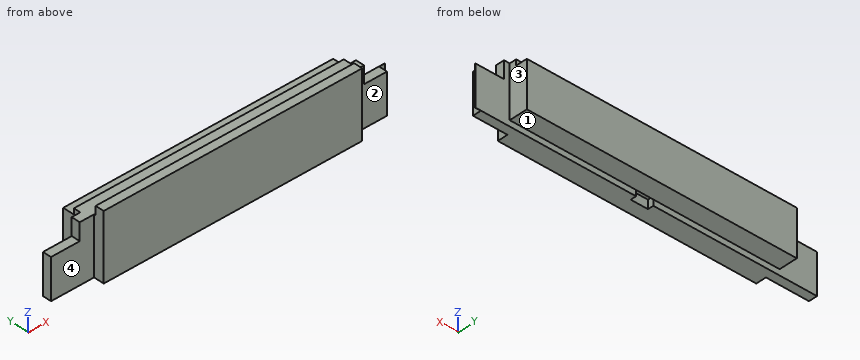
from build123d import *

# Parameters (mm, degrees)
SKETCH042_W     = 610
SKETCH042_H     = 115
PAD004_DEPTH    = 65
SKETCH043_W     = 60
SKETCH043_H     = 32
SKETCH043_W_2   = 70
SKETCH043_H_2   = 18
POCKET037_DEPTH = 115.001
SKETCH044_W     = 80
SKETCH044_H     = 32
SKETCH044_W_2   = 90
SKETCH044_H_2   = 18
POCKET038_DEPTH = 115.001
SKETCH045_W     = 50
SKETCH045_H     = 45
POCKET039_DEPTH = 65.001
SKETCH046_W     = 65
SKETCH046_H     = 45
POCKET040_DEPTH = 65.001
SKETCH047_W     = 30
SKETCH047_H     = 10
POCKET041_DEPTH = 15
SKETCH048_W     = 610
SKETCH048_H     = 32
POCKET042_DEPTH = 10
SKETCH049_W     = 20
SKETCH049_H     = 25
POCKET043_DEPTH = 610.001
SKETCH050_W     = 50
SKETCH050_H     = 15
POCKET044_DEPTH = 610.001
SKETCH051_W     = 15
SKETCH051_H     = 65
POCKET045_DEPTH = 115.001
SKETCH052_W     = 10
SKETCH052_H     = 32.5
POCKET046_DEPTH = 115.001


with BuildPart() as part:
    # Sketch042 (on DatumPlane) → Pad004 (new body)
    with BuildSketch(Plane.XZ.offset(32.5)):
        Rectangle(SKETCH042_W, SKETCH042_H)
    extrude(amount=-PAD004_DEPTH)

    # Sketch043 (on DatumPlane) → Pocket037 (cut, through all)
    with BuildSketch(Plane.XY.offset(57.5)):
        with Locations((275, 16.5)):
            Rectangle(SKETCH043_W, SKETCH043_H)
        with Locations((270, -23.5)):
            Rectangle(SKETCH043_W_2, SKETCH043_H_2)
    extrude(amount=-POCKET037_DEPTH, mode=Mode.SUBTRACT)

    # Sketch044 (on DatumPlane) → Pocket038 (cut, through all)
    with BuildSketch(Plane.XY.offset(57.5)):
        with Locations((-265, 16.5)):
            Rectangle(SKETCH044_W, SKETCH044_H)
        with Locations((-260, -23.5)):
            Rectangle(SKETCH044_W_2, SKETCH044_H_2)
    extrude(amount=-POCKET038_DEPTH, mode=Mode.SUBTRACT)

    # Sketch045 (on DatumPlane) → Pocket039 (cut, through all)
    with BuildSketch(Plane.XZ.offset(32.5)):
        with Locations((280, 35)):
            Rectangle(SKETCH045_W, SKETCH045_H)
    extrude(amount=-POCKET039_DEPTH, mode=Mode.SUBTRACT)

    # Sketch046 (on DatumPlane) → Pocket040 (cut, through all)
    with BuildSketch(Plane.XZ.offset(32.5)):
        with Locations((-272.5, 35)):
            Rectangle(SKETCH046_W, SKETCH046_H)
    extrude(amount=-POCKET040_DEPTH, mode=Mode.SUBTRACT)

    # Sketch047 (on DatumPlane) → Pocket041 (cut)
    with BuildSketch(Plane(origin=(0, 0, -57.5), x_dir=(-1, 0, 0), z_dir=(0, 0, -1))):
        with Locations((-10, -4.5)):
            Rectangle(SKETCH047_W, SKETCH047_H)
    extrude(amount=-POCKET041_DEPTH, mode=Mode.SUBTRACT)

    # Sketch048 (on DatumPlane) → Pocket042 (cut)
    with BuildSketch(Plane(origin=(0, 0, -57.5), x_dir=(-1, 0, 0), z_dir=(0, 0, -1))):
        with Locations((0, 16.5)):
            Rectangle(SKETCH048_W, SKETCH048_H)
    extrude(amount=-POCKET042_DEPTH, mode=Mode.SUBTRACT)

    # Sketch049 (on DatumPlane) → Pocket043 (cut, through all)
    with BuildSketch(Plane.YZ.offset(305)):
        with Locations((22.5, 45)):
            Rectangle(SKETCH049_W, SKETCH049_H)
    extrude(amount=-POCKET043_DEPTH, mode=Mode.SUBTRACT)

    # Sketch050 (on DatumPlane) → Pocket044 (cut, through all)
    with BuildSketch(Plane.YZ.offset(305)):
        with Locations((7.5, 50)):
            Rectangle(SKETCH050_W, SKETCH050_H)
    extrude(amount=-POCKET044_DEPTH, mode=Mode.SUBTRACT)

    # Sketch051 (on DatumPlane) → Pocket045 (cut, through all)
    with BuildSketch(Plane.XY.offset(57.5)):
        with Locations((-297.5, 0)):
            Rectangle(SKETCH051_W, SKETCH051_H)
    extrude(amount=-POCKET045_DEPTH, mode=Mode.SUBTRACT)

    # Sketch052 (on DatumPlane) → Pocket046 (cut, through all)
    with BuildSketch(Plane.XY.offset(57.5)):
        with Locations((300, -16.25)):
            Rectangle(SKETCH052_W, SKETCH052_H)
    extrude(amount=-POCKET046_DEPTH, mode=Mode.SUBTRACT)


solid = part.part
Can you work these out from the model? Positions are in its coordinate system, mm. Face numbers are marked on the shaded views. A direction names the side the tool comes from. Give positions to 0.01 mm unless a question says otherwise; leave off trailing zeros. Loops run counter-clockwise (first coordinate to the right, second up) from the corner with the lowest first, then second, coordinate; pieces in that order, holes last. Notation, with made-up numbers: (33.5, 6.25) -> (45.5, 6.25) arc R9 ccw to (45.5, 21.25) -> close; hole circle Ø7 at (25, 4.25). An arc over 180 degrees is marked (long way). Write item = value, one per line.
1) Will these pins go through, and if not, where does the flat tip stop? pin 1 (4 mm diameter, centred on x = -219.5, y = 21.5, fed in from -Z); pin 2 (5 mm diameter, centred on x = 13, y = -4, fed in from -Z); pin 3 (14.5 mm diameter, centred on y = -25, z = 6, fed in from +X).
Check result:
pin_1 = -47.5
pin_2 = -42.5
pin_3 = 235
2) Suppose I cut it at C-C on x = 6.5. Write out the boundary of the cut face in (y, z), then the cut area to 4 significant figures.
Check result:
outline = (-32.5, -57.5) -> (-9.5, -57.5) -> (-9.5, -42.5) -> (0.5, -42.5) -> (0.5, -47.5) -> (32.5, -47.5) -> (32.5, 32.5) -> (12.5, 32.5) -> (12.5, 42.5) -> (-17.5, 42.5) -> (-17.5, 57.5) -> (-32.5, 57.5) -> close
area = 6,055 mm2
3) Suppose I cut it at D-D on z = 27. Write out the boundary of the cut face in (x, y), then the cut area to 3 significant figures.
Check result:
outline = (-240, -14.5) -> (-215, -14.5) -> (-215, -32.5) -> (235, -32.5) -> (235, -14.5) -> (255, -14.5) -> (255, 0.5) -> (245, 0.5) -> (245, 32.5) -> (-225, 32.5) -> (-225, 0.5) -> (-240, 0.5) -> close
area = 30,600 mm2
4) Suppose I cut it at B-B on x = -73. Write out the boundary of the cut face in (y, z).
Check result:
outline = (-32.5, -57.5) -> (0.5, -57.5) -> (0.5, -47.5) -> (32.5, -47.5) -> (32.5, 32.5) -> (12.5, 32.5) -> (12.5, 42.5) -> (-17.5, 42.5) -> (-17.5, 57.5) -> (-32.5, 57.5) -> close
5) For the marked faces 1, 2, 3 and 4, which set-ups out of +Z, -Z, +X, -X, +Y, -Y let a thin tool reach every point of the face, with its end or its side?
Check result:
face_1 = -Z, +X, -X, +Y
face_2 = +Z, -Z, +X, -Y
face_3 = +Z, -Z, +X, +Y
face_4 = +Z, -Z, -X, -Y
6) Suppose I cut it at A-A on z = 2.5. Write out the boundary of the cut face in (x, y), then the cut area to 3 significant figures.
Check result:
outline = (-290, -14.5) -> (-215, -14.5) -> (-215, -32.5) -> (235, -32.5) -> (235, -14.5) -> (295, -14.5) -> (295, 0) -> (305, 0) -> (305, 0.5) -> (245, 0.5) -> (245, 32.5) -> (-225, 32.5) -> (-225, 0.5) -> (-290, 0.5) -> close
area = 31,900 mm2
7) I need wall thicknesses on L1, parallel to X at y = -3, z = -46.5; L2, parallel to Y at x = 203, z = 51; L3, parallel to X at y = 26.5, z = -36. Which ranges of each line are inside material? Lowest first, please. Write a range as from..to.
Check result:
L1 = -290..-5, 25..295
L2 = -32.5..-17.5
L3 = -225..245
